Read the model definition and answer for the solid it produces. Units are mm, in the model's axes. Round coordinates to 2 decimals unless told otherwise and drop trailing zeros. Loops run counter-clockwise (first coordinate to the right, second up) from the corner with the lowest first, then second, coordinate; pieces in that order, holes last. Notation, with made-up numbers: M 30.25,-0.5 L 58.25,-0.5 A23 cw 58.25,32.5 Z; hole C -18,89.25 d5. An arc over 180 degrees is marked long. Answer as CSV lines item,"result".
```python
from build123d import *

# Parameters (mm, degrees)
CROQUIS1_R              = 10
SALIENTE_EXTRUIR1_DEPTH = 10


with BuildPart() as part:
    # Croquis1 → Saliente-Extruir1 (new body)
    with BuildSketch(Plane.XY):
        Polygon((-53.033008589, 0), (0, 53.033008589), (53.033008589, 0), (0, -53.033008589), align=None)
        Circle(CROQUIS1_R, mode=Mode.SUBTRACT)
    extrude(amount=SALIENTE_EXTRUIR1_DEPTH)


solid = part.part
```
1) Find section D-D, the plane x = -27.5. Give the vertices of the cut face in (y, z).
Evaluation:
outline,"M -25.53,0 L 25.53,0 L 25.53,10 L -25.53,10 Z"
2) Determine the mould class of faces 1 (the flat face through (-26.888, 26.145, 4.93)), 2 (the cylindrical face through (-2.17, -9.76, 4.93)), 3 (the flat face through (1, 13, 10)) for opening direction Y: released by +Y, released by -Y, zero draft, split by the parting line, or undercut.
Evaluation:
face 1,"released by +Y"
face 2,"undercut"
face 3,"zero draft"
3) Find section C-C, the plane y = 19. Give the vertices of the cut face in (x, z), then the cut area to 3 significant figures.
Evaluation:
outline,"M -34.03,0 L 34.03,0 L 34.03,10 L -34.03,10 Z"
area,"681 mm^2"
4) Find section A-A, the plane z = 5.75. Give the vertices of the cut face in (x, y).
Evaluation:
outline,"M -53.03,0 L 0,-53.03 L 53.03,0 L 0,53.03 Z; hole C 0,0 d20"
5) Find section B-B, the plane y = -6.5. Give the vertices of the cut face in (x, z).
Evaluation:
outline,"M -46.53,0 L -7.6,0 L -7.6,10 L -46.53,10 Z; M 7.6,0 L 46.53,0 L 46.53,10 L 7.6,10 Z"
6) Straight lines are drawn through the part: line 1 (Y direction, x = 0, z = 7); line 2 (X direction, y = -1, z = 0.5); line 3 (X direction, y = -9, z = 9.5). For each, find the intervals that lie inside material, in ascending order.
Evaluation:
line 1,"y = -53.03 to -10, 10 to 53.03"
line 2,"x = -52.03 to -9.95, 9.95 to 52.03"
line 3,"x = -44.03 to -4.36, 4.36 to 44.03"
7) Each of these flat-tipped pins is pushed along its axis until it touches: P1, Ø1.5, axis at x = -10.5, z = 1, coming from the -Y side; P2, Ø10, axis at x = -18, y = -20.5, coming from the -Z side; P3, Ø18, axis at x = 0, y = 0, coming from the +Z side; P4, Ø3, axis at y = -11, z = 1, coming from the +X side. Where does it stop, or does it pass through?
Evaluation:
P1,"stops at y = -43.28"
P2,"stops at z = 0"
P3,"passes through"
P4,"stops at x = 43.53"
